Read the model definition and answer for the solid it produces. Units are mm, in the model's axes. Face numbers are marked on the shaded views. Give positions to 0.01 mm unless a question says otherwise; leave off trailing zeros. Loops run counter-clockwise (first coordinate to the right, second up) from the corner with the lowest first, then second, coordinate; pieces in that order, holes last. Notation, with made-up numbers: (-30, -7) - (-2, -7) arc R21 ccw to (-2, 31) - close; hole circle Ø6 at (47.25, 81). An arc over 180 degrees is marked (long way). Write item = value, one per line. Start each with the question number.
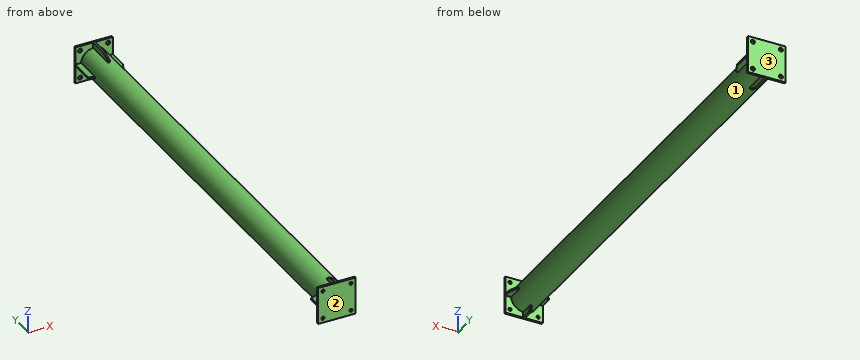
from build123d import *

# Parameters (mm, degrees)
F0_R          = 70
F0_R_2        = 65
F1_DEPTH      = 2434
F2_W          = 200
F2_H          = 200
F2_R          = 11
F3_DEPTH      = 10
F4_W          = 30.1787997812
F4_H          = 10
F4_W_2        = 10
F4_H_2        = 30.1787997812
F5_DEPTH      = 150
F6_T1_DEPTH   = 269.311363913
F6_T3_DEPTH   = 269.311363913
F6_T8_DEPTH   = 269.311363913
F6_S9_R       = 70
F6_T10_DEPTH  = 139
F8_W          = 200
F8_H          = 200
F8_R          = 8.5
F9_DEPTH      = 10
F10_W         = 10
F10_H         = 30.1787997812
F10_W_2       = 30.1787997812
F10_H_2       = 10
F11_DEPTH     = 80
F12_T1_DEPTH  = 269.311363913
F12_T3_DEPTH  = 269.311363913
F12_T8_DEPTH  = 269.311363913
F12_S9_R      = 70
F12_T10_DEPTH = 139
F12_T14_DEPTH = 269.311363913
F12_S15_R     = 70
F12_T16_DEPTH = 139


# Not quite as in the source:
# - a fillet or chamfer that OpenCascade refuses, or shapes differently, is made with other operations: its cross-section is extruded or revolved along the edge and cut away or added


with BuildPart() as f1:
    # F0 (on Front) → F1 (new body)
    with BuildSketch(Plane.XZ):
        Circle(F0_R)
        Circle(F0_R_2, mode=Mode.SUBTRACT)
    extrude(amount=F1_DEPTH)

    # F2 (on Front) → F3 (join)
    with BuildSketch(Plane.XZ):
        Rectangle(F2_W, F2_H)
        with Locations((-75, -75)):
            Circle(F2_R, mode=Mode.SUBTRACT)
        with Locations((75, -75)):
            Circle(F2_R, mode=Mode.SUBTRACT)
        with Locations((-75, 75)):
            Circle(F2_R, mode=Mode.SUBTRACT)
        with Locations((75, 75)):
            Circle(F2_R, mode=Mode.SUBTRACT)
    extrude(amount=-F3_DEPTH)

    # F4 (on Front) → F5 (join)
    with BuildSketch(Plane.XZ):
        with Locations((-84.9106001094, 0)):
            Rectangle(F4_W, F4_H)
        with Locations((0, 84.9106001094)):
            Rectangle(F4_W_2, F4_H_2)
        with Locations((84.9106001094, 0)):
            Rectangle(F4_W, F4_H)
        with Locations((0, -84.9106001094)):
            Rectangle(F4_W_2, F4_H_2)
    extrude(amount=F5_DEPTH)

    # F6: chamfer of 50 x 20 on 4 edges, made by hand

    # F6_s2 → F6_t1 (cut)
    with BuildSketch(Plane.YZ.offset(-134.6556819565)):
        Polygon((-100, 100), (-150, 80), (-150, 100), align=None)
        Polygon((-100, -100), (-150, -80), (-150, -100), align=None)
    extrude(amount=F6_T1_DEPTH, mode=Mode.SUBTRACT)

    # F6_s4 → F6_t3 (cut)
    with BuildSketch(Plane.XY.offset(-134.6556819565)):
        Polygon((100, -100), (80, -150), (100, -150), align=None)
    extrude(amount=F6_T3_DEPTH, mode=Mode.SUBTRACT)


with BuildPart() as f6_tool6:
    # F6_s7 → F6_t8 (new body)
    with BuildSketch(Plane.XY.offset(134.6556819565)):
        Polygon((-100, -130), (-50, -150), (-100, -150), align=None)
    extrude(amount=-F6_T8_DEPTH)

    # F6_s9 → F6_t10 (cut, symmetric)
    with BuildSketch(Plane.XZ.offset(140)):
        Circle(F6_S9_R)
    extrude(amount=F6_T10_DEPTH, both=True, mode=Mode.SUBTRACT)


with BuildPart() as f1_1:
    add(f1.part)

    # F6_t5: cut F6_tool6
    add(f6_tool6.part, mode=Mode.SUBTRACT)

    # F8 (on offset) → F9 (join)
    with BuildSketch(Plane.XZ.offset(2434)):
        Rectangle(F8_W, F8_H)
        with Locations((-75, -75)):
            Circle(F8_R, mode=Mode.SUBTRACT)
        with Locations((75, -75)):
            Circle(F8_R, mode=Mode.SUBTRACT)
        with Locations((-75, 75)):
            Circle(F8_R, mode=Mode.SUBTRACT)
        with Locations((75, 75)):
            Circle(F8_R, mode=Mode.SUBTRACT)
    extrude(amount=F9_DEPTH)

    # F10 (on face) → F11 (join)
    with BuildSketch(Plane(origin=(0, -2434, 0), x_dir=(-1, 0, 0), z_dir=(0, 1, 0))):
        with Locations((0, 84.9106001094)):
            Rectangle(F10_W, F10_H)
        with Locations((84.9106001094, 0)):
            Rectangle(F10_W_2, F10_H_2)
        with Locations((0, -84.9106001094)):
            Rectangle(F10_W, F10_H)
        with Locations((-84.9106001094, 0)):
            Rectangle(F10_W_2, F10_H_2)
    extrude(amount=F11_DEPTH)

    # F12: chamfer of 20 x 50 on 4 edges, made by hand

    # F12_s2 → F12_t1 (cut)
    with BuildSketch(Plane.YZ.offset(-134.6556819565)):
        Polygon((-2404, 100), (-2354, 80), (-2354, 100), align=None)
    extrude(amount=F12_T1_DEPTH, mode=Mode.SUBTRACT)

    # F12_s4 → F12_t3 (cut)
    with BuildSketch(Plane.XY.offset(-134.6556819565)):
        Polygon((100, -2404), (80, -2354), (100, -2354), align=None)
    extrude(amount=F12_T3_DEPTH, mode=Mode.SUBTRACT)


with BuildPart() as f12_tool6:
    # F12_s7 → F12_t8 (new body)
    with BuildSketch(Plane.XY.offset(-134.6556819565)):
        Polygon((-100, -2374), (-50, -2354), (-100, -2354), align=None)
    extrude(amount=F12_T8_DEPTH)

    # F12_s9 → F12_t10 (cut, symmetric)
    with BuildSketch(Plane.XZ.offset(2364)):
        Circle(F12_S9_R)
    extrude(amount=F12_T10_DEPTH, both=True, mode=Mode.SUBTRACT)


with BuildPart() as f1_2:
    add(f1_1.part)

    # F12_t5: cut F12_tool6
    add(f12_tool6.part, mode=Mode.SUBTRACT)


with BuildPart() as f12_tool12:
    # F12_s13 → F12_t14 (new body)
    with BuildSketch(Plane.YZ.offset(134.6556819565)):
        Polygon((-2374, -100), (-2354, -50), (-2354, -100), align=None)
    extrude(amount=-F12_T14_DEPTH)

    # F12_s15 → F12_t16 (cut, symmetric)
    with BuildSketch(Plane.XZ.offset(2364)):
        Circle(F12_S15_R)
    extrude(amount=F12_T16_DEPTH, both=True, mode=Mode.SUBTRACT)


with BuildPart() as f1_3:
    add(f1_2.part)

    # F12_t11: cut F12_tool12
    add(f12_tool12.part, mode=Mode.SUBTRACT)


solid = f1_3.part
1. For a pull along Y with two mould halves and no side action, classify the marked faces 1, 2 and 3 as released by +Y, released by -Y, zero draft, split by the parting line, or undercut.
2. Consider line 1 along Z through (x, y) = (-75, 5.25); line 2 along Y through (x, z) = (59, -26.5); line 3 along Z through (x, y) = (-75, -2437). Determine where each line is inside the solid, lowest interval first. Write a range as [from, to].
3. Given P1, Ø4, axis at x = 65, y = -298.5, coming from the +Z side; P2, Ø13, axis at x = -75, z = -75, coming from the +Y side; P3, Ø15, axis at x = 87.5, y = -2391, coming from the -Z side; P4, Ø4, axis at x = -10.5, y = -1690.5, coming from the +Z side, each flat-ended and moving along its own axis, determine where each tip first touches the part or whether it passes through.
4. A cutting plane is placed at B-B on y = -609.5. Give the vertices of the cut face in (x, z).
5. A cutting plane is placed at A-A on x = 42. Give the vertices of the cut face in (y, z), and give its area (3 significant figures).
Reply:
q1.face_1 = undercut
q1.face_2 = released by -Y
q1.face_3 = released by +Y
q2.line_1 = [-100, -86], [-64, 64], [86, 100]
q2.line_2 = [-2444, -2434], [0, 10]
q2.line_3 = [-100, -83.5], [-66.5, 66.5], [83.5, 100]
q3.P1 = 30.51
q3.P2 = through
q3.P3 = -5
q3.P4 = 69.48
q4.outline = circle Ø140 at (0, 0); hole circle Ø130 at (0, 0)
q5.outline = (-2444, -100) - (-2434, -100) - (-2434, -56) - (0, -56) - (0, -100) - (10, -100) - (10, 100) - (0, 100) - (0, 56) - (-2434, 56) - (-2434, 100) - (-2444, 100) - close; hole (-2434, -49.61) - (0, -49.61) - (0, 49.61) - (-2434, 49.61) - close
q5.area = 35,100 mm^2
